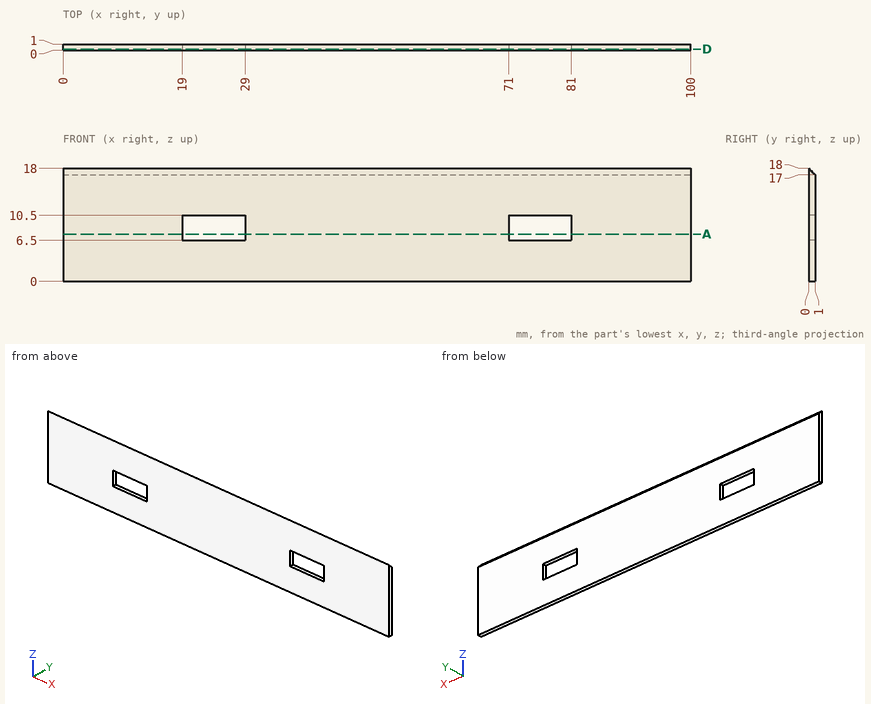
Study the drawing (mm; zero at the part's minimum x, y, z) and answer. Give positions to 0.01 mm unless a question says otherwise; leave off trailing zeros. Write each loop counter-clockwise with the first axis right and the second up, starting at its lowest first coordinate (ties: lowest second). Pieces come first, ordered by that corner, then holes.
Item 1: Section D-D, the plane y = 0.2 is taken. Write down the section's boundary in (x, z), plus the area to 3 significant figures.
Item 2: A flat-ended cylindrical pin translates along its axis: P1, Ø0.5, axis at x = 74.5, y = 0.5, coming from the +Z side. Find the tip coordinate at first contact, or state that the pin passes through.
Item 3: Section A-A, the plane z = 7.5 is taken. Write down the section's boundary in (x, y), plus the area to 3 significant figures.
Item 4: Find the intervals of material crossed by line 1 along X through (y, z) = (0.3, 8); line 2 along Z through (x, y) = (27.5, 0.9); line 3 along Z through (x, y) = (29.5, 0.9), in increasing order.
Completed:
1. outline: (0, 0) - (100, 0) - (100, 17.8) - (0, 17.8) - close; hole (19, 6.5) - (29, 6.5) - (29, 10.5) - (19, 10.5) - close; hole (71, 6.5) - (81, 6.5) - (81, 10.5) - (71, 10.5) - close
1. area: 1,700 mm2
2. P1: stops at z = 17.75
3. outline: (0, 0) - (19, 0) - (19, 1) - (0, 1) - close; (29, 0) - (71, 0) - (71, 1) - (29, 1) - close; (81, 0) - (100, 0) - (100, 1) - (81, 1) - close
3. area: 80.0 mm2
4. line 1: x = 0 to 19, 29 to 71, 81 to 100
4. line 2: z = 0 to 6.5, 10.5 to 17.1
4. line 3: z = 0 to 17.1
